```python
from build123d import *

# Parameters (mm, degrees)
SALIENTE_EXTRUIR1_DEPTH = 4
CROQUIS2_W              = 6.75
CROQUIS2_H              = 5
SALIENTE_EXTRUIR2_DEPTH = 18
CROQUIS3_R              = 2
CORTAR_EXTRUIR1_DEPTH   = 10
SALIENTE_EXTRUIR3_DEPTH = 5
CROQUIS6_W              = 25
CROQUIS6_H              = 3
SALIENTE_EXTRUIR4_DEPTH = 20
CROQUIS7_R              = 7.5
SALIENTE_EXTRUIR5_DEPTH = 8
CORTAR_EXTRUIR2_DEPTH   = 3
CORTAR_EXTRUIR3_REACH   = 6
CROQUIS9_W              = 16
CROQUIS9_H              = 9
CHAFL_N1_SIZE           = 3


with BuildPart() as part:
    # Croquis1 → Saliente-Extruir1 (new body)
    with BuildSketch(Plane(origin=(0, 0, 0), x_dir=(1, 0, 0), z_dir=(0, 1, 0))):
        Polygon((12.331887662, -35.204744953), (33.9207519, -13.615880715), (33.9207519, 29.795255047), (-40.0792481, 29.795255047), (-40.0792481, -35.204744953), align=None)
    extrude(amount=SALIENTE_EXTRUIR1_DEPTH)

    # Croquis2 → Saliente-Extruir2 (add)
    with BuildSketch(Plane(origin=(0, 4, 0), x_dir=(1, 0, 0), z_dir=(0, 1, 0))):
        with Locations((-21.9542481, -10)):
            Rectangle(CROQUIS2_W, CROQUIS2_H)
        with Locations((25.7957519, -10)):
            Rectangle(CROQUIS2_W, CROQUIS2_H)
    extrude(amount=SALIENTE_EXTRUIR2_DEPTH)

    # Croquis3 → Cortar-Extruir1 (cut)
    with BuildSketch(Plane.XY.offset(12.5)):
        with Locations((-22.2292481, 9)):
            Circle(CROQUIS3_R)
        with Locations((-22.2292481, 19)):
            Circle(CROQUIS3_R)
        with Locations((26.0707519, 19)):
            Circle(CROQUIS3_R)
        with Locations((26.0707519, 9)):
            Circle(CROQUIS3_R)
    extrude(amount=-CORTAR_EXTRUIR1_DEPTH, mode=Mode.SUBTRACT)

    # Croquis5 → Saliente-Extruir3 (add)
    with BuildSketch(Plane.XY.offset(12.5)):
        with BuildLine():
            Line((-25.3292481, 4), (-25.3292481, 22))
            Line((-25.3292481, 22), (-18.5792481, 22))
            Line((-18.5792481, 22), (-18.5792481, 27.393443103))
            Line((-18.5792481, 27.393443103), (-23.831494252, 27.393443103))
            ThreePointArc((-23.831494252, 27.393443103), (-27.046864835, 15.854637612), (-25.3292481, 4))
        make_face()
        with BuildLine():
            Line((29.1707519, 4), (29.1707519, 22))
            Line((29.1707519, 22), (22.4207519, 22))
            Line((22.4207519, 22), (22.4207519, 27.393443103))
            Line((22.4207519, 27.393443103), (27.672998052, 27.393443103))
            ThreePointArc((27.672998052, 27.393443103), (30.888368635, 15.854637612), (29.1707519, 4))
        make_face()
    extrude(amount=-SALIENTE_EXTRUIR3_DEPTH)

    # Croquis6 → Saliente-Extruir4 (add)
    with BuildSketch(Plane(origin=(0, 4, 0), x_dir=(1, 0, 0), z_dir=(0, 1, 0))):
        with Locations((12.0707519, 26)):
            Rectangle(CROQUIS6_W, CROQUIS6_H)
    extrude(amount=SALIENTE_EXTRUIR4_DEPTH)

    # Croquis7 → Saliente-Extruir5 (add)
    with BuildSketch(Plane(origin=(0, 0, -27.5), x_dir=(-1, 0, 0), z_dir=(0, 0, -1))):
        with Locations((-12.0707519, 14)):
            Circle(CROQUIS7_R)
    extrude(amount=SALIENTE_EXTRUIR5_DEPTH)

    # Croquis8 → Cortar-Extruir2 (cut)
    with BuildSketch(Plane(origin=(0, 0, -27.5), x_dir=(-1, 0, 0), z_dir=(0, 0, -1))):
        with BuildLine():
            Line((-24.5707519, 24), (-24.5707519, 4))
            Line((-24.5707519, 4), (-22.0707519, 14))
            ThreePointArc((-22.0707519, 14), (-19.141819712, 21.071067812), (-12.0707519, 24))
            Line((-12.0707519, 24), (-24.5707519, 24))
        make_face()
        with BuildLine():
            Line((0.4292481, 24), (-12.0707519, 24))
            ThreePointArc((-12.0707519, 24), (-4.999684088, 21.071067812), (-2.0707519, 14))
            Line((-2.0707519, 14), (0.4292481, 4))
            Line((0.4292481, 4), (0.4292481, 24))
        make_face()
    extrude(amount=-CORTAR_EXTRUIR2_DEPTH, mode=Mode.SUBTRACT)

    # Croquis9 → Cortar-Extruir3 (cut, up to next)
    with BuildSketch(Plane(origin=(0, 4, 0), x_dir=(1, 0, 0), z_dir=(0, 1, 0)), mode=Mode.PRIVATE) as cortar_extruir3_sk1:
        with Locations((12.4207519, -25)):
            Rectangle(CROQUIS9_W, CROQUIS9_H)
    cortar_extruir3_tool1 = extrude(cortar_extruir3_sk1.sketch, amount=-CORTAR_EXTRUIR3_REACH, mode=Mode.PRIVATE) & part.part
    add(cortar_extruir3_tool1.solids().sort_by_distance((12.420752, 4, 25))[0], mode=Mode.SUBTRACT)

    # Chaflán1
    chafl_n1_edges = [part.edges().sort_by_distance(p)[0] for p in [
        (33.9207519, 0, -8.089687166),
    ]]
    chamfer(chafl_n1_edges, length=CHAFL_N1_SIZE)


solid = part.part
```
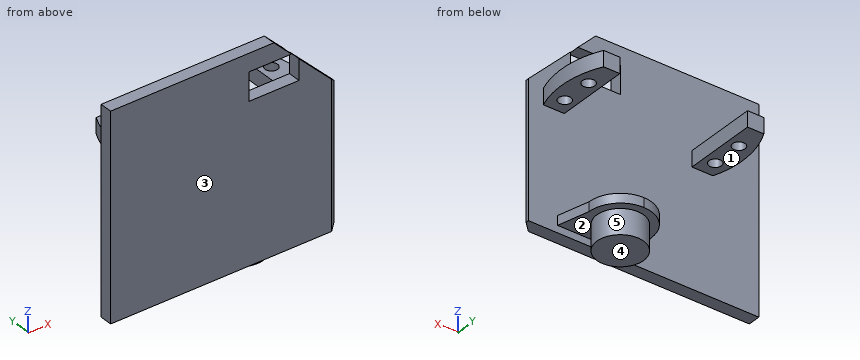
Model file for the job. Use its own axes, mm. Face numbers are marked on the shaded views. A direction names the side the tool comes from. Coordinates: 2 decimals unless noted, no trailing zeros. Write each loop counter-clockwise with the first axis right and the second up, starting at its lowest first coordinate (ties: lowest second). Pieces come first, ordered by that corner, then holes. Notation, with made-up numbers: (31.25, 30.5) - (61.25, 30.5) arc R27 cw to (61.25, 51.5) - close; hole circle Ø11 at (54.5, 72.5). An arc over 180 degrees is marked (long way). Use a Markdown table: item, result. Add a question column.
Item 1: Drill centre lines: line 1 along Z through (x, y) = (9.5, 19.75); line 2 along Y through (x, z) = (9.5, -3); line 3 along Z through (x, y) = (28.5, 7.25). Where is each one in solid material? Low to high.
Item 2: Band-saw the part on D-D, the plane x = -32. Write the cut outline in (y, z), and give its area (3 significant figures).
Item 3: Band-saw the part on B-B, the plane y = 25.75. Write the cut outline in (x, z).
Item 4: Band-saw the part on A-A, the plane z = -12. Write the cut outline in (x, y).
Item 5: Two-plate mould, pull along Y, no slides. Class the marked faces 1, 2 and 3: pulls with the +Y half, pulls with the -Y half, needs draft (parallel to the pull), parting line crosses it, or undercut.
Item 6: 3-axis set-ups, long thin cutter, end or side, ignore diameter. For the marked faces 4 and 5: which of +Z, -Z, +X, -X, +Y, -Y reach the whole face in a straight line?
Item 7: Drop flat-ended pins along their axis: pin 1 (5 mm diameter, centred on x = 26.07, y = 19, fed in from -Z); pin 2 (12 mm diameter, centred on y = 13.5, z = 22.5, fed in from +X); pin 3 (2 mm diameter, centred on x = 22.5, z = 15, fed in from +Y); pin 4 (3 mm diameter, centred on x = -7, y = 3, fed in from -Z). Give the stop position or say it passes through.
Item 8: Band-saw the part on C-C, the plane y = 9. Write the cut outline in (x, z), and give its area (3 significant figures).
A:
| question | item | result |
|---|---|---|
| 1 | line 1 | z = -35.5 to -24.5 |
| 1 | line 2 | y = 0 to 4 |
| 1 | line 3 | z = 7.5 to 12.5 |
| 2 | outline | (0, -29.8) - (4, -29.8) - (4, 35.2) - (0, 35.2) - close |
| 2 | area | 260 mm² |
| 3 | outline | (-24.62, 7.5) - (-18.58, 7.5) - (-18.58, 12.5) - (-24.62, 12.5) - close; (22.42, 7.5) - (28.46, 7.5) - (28.46, 12.5) - (22.42, 12.5) - close |
| 4 | outline | (-40.08, 0) - (30.92, 0) - (33.92, 3) - (33.92, 4) - (-40.08, 4) - close |
| 5 | face 1 | needs draft |
| 5 | face 2 | undercut |
| 5 | face 3 | pulls with the -Y half |
| 6 | face 4 | -Z, +X, -X, +Y, -Y |
| 6 | face 5 | -Z |
| 7 | pin 1 | stops at z = 7.5 |
| 7 | pin 2 | passes through |
| 7 | pin 3 | stops at y = 4 |
| 7 | pin 4 | stops at z = -29.8 |
| 8 | outline | (-26.67, 7.5) - (-24.23, 7.5) - (-24.23, 12.5) - (-26.67, 12.5) - close; (-20.23, 7.5) - (-18.58, 7.5) - (-18.58, 12.5) - (-20.23, 12.5) - close; (0.82, -27.5) - (6.48, -27.5) - (6.48, -35.5) - (17.66, -35.5) - (17.66, -27.5) - (23.32, -27.5) - (23.32, -24.5) - (0.82, -24.5) - close; (22.42, 7.5) - (24.07, 7.5) - (24.07, 12.5) - (22.42, 12.5) - close; (28.07, 7.5) - (30.51, 7.5) - (30.51, 12.5) - (28.07, 12.5) - close |
| 8 | area | 198 mm² |
